Autodesk Inventor part; units mm, degrees
ref_plane "YZ Plane" through (0, 0, 0) normal (1, 0, 0) x (0, 1, 0)
ref_plane "XZ Plane" through (0, 0, 0) normal (0, 1, 0) x (-1, 0, 0)
ref_plane "XY Plane" through (0, 0, 0) normal (0, 0, 1) x (1, 0, 0)
sketch "Sketch1" plane through (0, 0, 0) normal (0, 0, 1) x (1, 0, 0)
  line L0 (4.25, 0) -> (4.25, 4.5)
  line L1 (4.25, 4.5) -> (0, 4.5)
  line L2 (4.25, 0) -> (1.75, 0)
  line L3 (1.75, 0) -> (1.75, -10)
  line L4 (1.75, -10) -> (2.5, -10)
  line L5 (2.5, -10) -> (2.5, -16)
  line L6 (2.5, -16) -> (0, -16)
  line L7 (0, 4.5) -> (0, -16)
  point P0 (0, 0)
  dimension "d0" = 8.5
  dimension "d2" = 3.5
  dimension "d3" = 5
  dimension "d4" = 4.5
  dimension "d5" = 6
  dimension "d6" = 16
revolve "Вращение1" add sketch "Sketch1" angle 360 about axis through (0, 4.5, 0) along (0, -1, 0)
sketch "Sketch2" plane through (0, 4.5, 0) normal (0, 1, 0) x (1, 0, 0)
  circle A0 centre (0, 0) radius 4.25 construction
  circle A1 centre (0, 0) radius 1.25
  dimension "d31" = 2.5
extrude "Выдавливание1" cut sketch "Sketch2" against normal blind 1.5
chamfer "Фаска1" distance 0.9 angle 45 1 edges at (-4.25, 4.5, 0)
sketch "Sketch3" plane through (0, 0, 0) normal (0, 0, 1) x (1, 0, 0)
  line L0 (0, 0) -> (0, 4.5)
  line L1 (-2.3552, 0) -> (2.3552, 0) construction
  line L2 (-4.25, 4.5) -> (4.25, 4.5) construction
  line L3 (-0.6, 4.5) -> (0.6, 4.5)
  line L4 (0.6, 4.5) -> (0.6, 1.3)
  line L5 (0.6, 1.3) -> (-0.6, 1.3)
  line L6 (-0.6, 1.3) -> (-0.6, 4.5)
  dimension "d8" = 1.3
  dimension "d9" = 1.2
extrude "Выдавливание2" cut sketch "Sketch3" along normal through all both and the other way through all
fillet "Сопряжение1" radius 0.4 2 edges at (-1.75, 0, 0) (-1.75, -10, 0)
thread "Резьба1"
chamfer "Фаска2" distance 0.9 angle 45 1 edges at (-2.5, -16, 0)
equation "\"d31\" = d3_"
equation "\"d32\" = h3"
equation "\"d21\" = C1"
equation "\"d8\" = h2"
equation "\"d9\" = n"
equation "\"d12\" = R"
equation "\"d13\" = b"
equation "\"d15\" = C1"
equation "\"d0\" = D"
equation "\"d2\" = d1"
equation "\"d3\" = d_"
equation "\"d4\" = k1"
equation "\"d5\" = b"
equation "\"d6\" = l_"
equation "\"D\" = 8.5"
equation "\"d_\" = 5"
equation "\"l_\" = 16"
equation "\"b\" = 6"
equation "\"d1\" = 3.5"
equation "\"R\" = 0.4"
equation "\"C1\" = 0.9"
equation "\"h2\" = 1.3"
equation "\"n\" = 1.2"
equation "\"h3\" = 1.5"
equation "\"k1\" = 4.5"
equation "\"d3_\" = 2.5"
properties part number "Винт 3 M5-6gx16 ГОСТ 10336-80" material "Сталь, мягкая"
Part model, mm, in its own coordinate system. A direction names the side the tool comes from. Give positions to 0.01 mm unless a question says otherwise; leave off trailing zeros. Write each loop counter-clockwise with the first axis right and the second up, starting at its lowest first coordinate (ties: lowest second). Pieces come first, ordered by that corner, then holes. Notation, with made-up numbers: M -21.75,66.25 L 26.25,66.25 A11 cw 26.25,87.25 Z; hole C 62,81.25 d7. An arc over 180 degrees is marked long. Use CSV: the item, a comma, the result in double quotes.
Item 1: Slice it at B-B on z = 0. Write the cut outline in (x, y).
Taken from the geometry:
outline,"M -4.25,0 L -2.15,0 A0.4 cw -1.75,-0.4 L -1.75,-9.6 A0.4 cw -2.15,-10 L -2.5,-10 L -2.5,-15.1 L -1.6,-16 L 1.6,-16 L 2.5,-15.1 L 2.5,-10 L 2.15,-10 A0.4 cw 1.75,-9.6 L 1.75,-0.4 A0.4 cw 2.15,0 L 4.25,0 L 4.25,3.6 L 3.35,4.5 L 1.25,4.5 L 1.25,3 L 0.6,3 L 0.6,1.3 L -0.6,1.3 L -0.6,3 L -1.25,3 L -1.25,4.5 L -3.35,4.5 L -4.25,3.6 Z"
Item 2: Slice it at A-A on x = 0. Write the cut outline in (y, z), plus the area to 3 significant figures.
Taken from the geometry:
outline,"M -16,-1.6 L -15.1,-2.5 L -10,-2.5 L -10,-2.15 A0.4 cw -9.6,-1.75 L -0.4,-1.75 A0.4 cw 0,-2.15 L 0,-4.25 L 1.3,-4.25 L 1.3,4.25 L 0,4.25 L 0,2.15 A0.4 cw -0.4,1.75 L -9.6,1.75 A0.4 cw -10,2.15 L -10,2.5 L -15.1,2.5 L -16,1.6 Z"
area,"75.4 mm²"
Item 3: Which spindle directions (+Z, -Z, +X, -X, +Y, -Y) get a long thin tool onto all of the face, cutting with end or side? Do faces 5 (the face through (-2, 4.5, 0)), 6 (the face through (0.6, 2.6, -0.1)), 7 (the face through (1.617, -5.064, -0.67)), 8 (the face through (1.25, 3.76, 0.02)). Say none if no direction does.
Taken from the geometry:
face 5,"+Z, -Z, +X, -X, +Y"
face 6,"+Z, -Z, +Y"
face 7,"none"
face 8,"+Y"
Item 4: Pin check, flat tips, straight feed: P1, Ø1.5, axis at y = -6, z = -0.5, coming from the -X side; P2, Ø5, axis at y = -1, z = -3, coming from the +X side; P3, Ø3, axis at x = 1.5, z = -3.5, coming from the +Y side; P4, Ø1.5, axis at x = 2, y = -3.5, coming from the -Z side. Stop position of each tip, or through.
Taken from the geometry:
P1,"stops at x = -1.75"
P2,"stops at x = 4.19"
P3,"stops at y = 4.5"
P4,"stops at z = -1.22"
Item 5: Slice it at D-D on y = -12.75. Write the cut outline in (x, z), plus the area to 3 significant figures.
Taken from the geometry:
outline,"C 0,0 d5"
area,"19.6 mm²"
Item 6: Drill centre lines: probe 1 along Z at (x, y) = (0, -1.5); probe 2 along Y at (x, z) = (-1.75, 0.5); probe 3 along Y at (x, z) = (-1, 2.75). Where is each one in solid material? Low to high.
Taken from the geometry:
probe 1,"z = -1.75 to 1.75"
probe 2,"y = -15.78 to -9.83, -0.17 to 4.5"
probe 3,"y = 0 to 4.5"
Item 7: Slice it at C-C on y = 1.75. Write the cut outline in (x, z), plus the area to 3 significant figures.
Taken from the geometry:
outline,"M -0.6,-4.21 L -0.6,4.21 A4.25 ccw Z; M 0.6,-4.21 A4.25 ccw 0.6,4.21 Z"
area,"46.6 mm²"
Item 8: Pull direction X, two halves, no side cores. Call faces 1 (the face through (-0.6, 2.5, -0.1)), 2 (the face through (-0.54, -12.59, -2.44)), 3 (the face through (-3.51, 4.34, 0.07)), 4 (the face through (0, 1.3, 0)): +X half, -X half, draft (parallel to the pull), parting line (faces both ways), or undercut.
Taken from the geometry:
face 1,"undercut"
face 2,"parting line"
face 3,"-X half"
face 4,"undercut"
